Autodesk Fusion 360 part; units mm, degrees
sketch "Sketch1" plane through (0, 0, 0) normal (0, 0, 1) x (1, 0, 0)
  line L0 (0, 0) -> (50, 0)
  line L1 (50, 0) -> (50, 30)
  line L2 (50, 30) -> (0, 30)
  line L3 (0, 30) -> (0, 0)
  dimension "d1" = 50
  dimension "d2" = 30
extrude "Extrude1" add sketch "Sketch1" along normal blind 30
sketch "Sketch2" plane through (0, 0, 30) normal (0, 0, 1) x (1, 0, 0)
  line L0 (0, 30) -> (0, 0)
  line L1 (0, 0) -> (50, 0)
  line L2 (50, 0) -> (50, 30)
  line L3 (50, 30) -> (0, 30)
  line L4 (0, 30) -> (0, 15)
  line L5 (0, 15) -> (10, 15)
  line L6 (0, 15) -> (25, 15)
  line L7 (50, 15) -> (40, 15)
  circle A0 centre (10, 15) radius 2.725
  circle A1 centre (40, 15) radius 2.725
  circle A2 centre (25, 15) radius 5.125
  dimension "d5" = 10
  dimension "d6" = 25
  dimension "d7" = 10
  dimension "d8" = 5.45
  dimension "d9" = 5.45
  dimension "d10" = 10.25
extrude "Extrude2" cut sketch "Sketch2" against normal blind 30 contours A2 | L5 L6 A0 | L5 L6 A0 | A1
sketch "Sketch3" plane through (0, 0, 0) normal (0, -1, 0) x (1, 0, 0)
  line L0 (0, 0) -> (50, 0)
  line L1 (50, 0) -> (50, 30)
  line L2 (50, 30) -> (0, 30)
  line L3 (0, 30) -> (0, 0)
  line L4 (50, 0) -> (50, 5)
  line L5 (50, 5) -> (25, 5)
  line L6 (25, 5) -> (25, 10)
  line L7 (25, 10) -> (50, 10)
  line L8 (50, 10) -> (50, 5)
  dimension "d13" = 5
  dimension "d14" = 25
  dimension "d15" = 5
extrude "Extrude3" cut sketch "Sketch3" against normal blind 5 contours L1 L5 L6 L7 L8
Here's how the part is built. I have some questions about the finished solid (model axes, mm). A direction names the side the tool comes from. Round coordinates to 2 decimals unless told otherwise and drop trailing zeros. Order: outer loops, then holes, each group sorted by start corner. A loop starts at its lowest first (then second) coordinate and runs counter-clockwise, first axis right, second up. Notation, with made-up numbers: M 33.25,17 L 72.25,17 A10 ccw 72.25,26 Z; hole C 77.25,42 d3. An arc over 180 degrees is marked long. Answer in a Markdown table with one row per item.
Item 1: For faces 1 (the face through (25, 0, 15)), 2 (the face through (37, 2, 10)), which set-ups out of +Z, -Z, +X, -X, +Y, -Y let a thin tool reach every point of the face, with its end or its side?
A:
| item | result |
|---|---|
| face 1 | +Z, -Z, +X, -X, -Y |
| face 2 | +X, -Y |
Item 2: Imagine slicing it at D-D, the plane y = 3.75. Write out the boundary of the cut face in (x, z).
A:
| item | result |
|---|---|
| outline | M 0,0 L 50,0 L 50,5 L 25,5 L 25,10 L 50,10 L 50,30 L 0,30 Z |
Item 3: Thinking about a two-plate mould opening in X: for faces 3 (the face through (25, 2, 7)), 4 (the face through (19, 15, 0)), 5 (the face through (27.36, 10.45, 15.21)), which applies, +X half, -X half, draft (parallel to the pull), parting line (faces both ways), or undercut?
A:
| item | result |
|---|---|
| face 3 | +X half |
| face 4 | draft |
| face 5 | undercut |
Item 4: Imagine slicing it at A-A, the plane x = 40. Write out the boundary of the cut face in (y, z) (3 decimals).
A:
| item | result |
|---|---|
| outline | M 0,0 L 12.275,0 L 12.275,30 L 0,30 L 0,10 L 5,10 L 5,5 L 0,5 Z; M 17.725,0 L 30,0 L 30,30 L 17.725,30 Z |
Item 5: Imagine slicing it at C-C, the plane y = 15. Write out the boundary of the cut face in (x, z) (3 decimals).
A:
| item | result |
|---|---|
| outline | M 0,0 L 7.275,0 L 7.275,30 L 0,30 Z; M 12.725,0 L 19.875,0 L 19.875,30 L 12.725,30 Z; M 30.125,0 L 37.275,0 L 37.275,30 L 30.125,30 Z; M 42.725,0 L 50,0 L 50,30 L 42.725,30 Z |
Item 6: Imagine slicing it at B-B, the plane z = 4. Write out the boundary of the cut face in (x, y) (3 decimals).
A:
| item | result |
|---|---|
| outline | M 0,0 L 50,0 L 50,30 L 0,30 Z; hole C 10,15 d5.45; hole C 25,15 d10.25; hole C 40,15 d5.45 |
Item 7: I'm going to push a flat-ended pin straight in: pin 1 (4 mm diameter, centred on x = 35.5, z = 7.5, fed in from -Y). Where does the tip first touch, or does it pass through?
A:
| item | result |
|---|---|
| pin 1 | stops at y = 5 |
Item 8: If I drill on L1, parallel to Y at x = 10, z = 6.75 (3 decimals); L2, parallel to X at y = 16.25, z = 28; L3, parallel to Y at x = 23, z = 13.5, over which ranges is the centre line in solid material (lowest first)? Write a range as from..to.
A:
| item | result |
|---|---|
| L1 | y = 0..12.275, 17.725..30 |
| L2 | x = 0..7.58, 12.42..20.03, 29.97..37.58, 42.42..50 |
| L3 | y = 0..10.28, 19.72..30 |
